The model under review builds one solid part; all positions refer to its coordinate system, in mm. Face numbers are marked on the shaded views. A direction names the side the tool comes from. Round coordinates to 2 decimals unless told otherwise and drop trailing zeros. Loops run counter-clockwise (first coordinate to the right, second up) from the corner with the lowest first, then second, coordinate; pieces in that order, holes last. Notation, with made-up numbers: M -27,0.5 L -1,0.5 A17 ccw -1,22.5 Z; hole C -36.5,-20.5 d11. An arc over 180 degrees is marked long. Answer as a JSON object with one key per item and string values. Group by question number.
Item 1: Tool access review of the marked faces 1 and 2: name each direction out of +Z, -Z, +X, -X, +Y, -Y from which nothing blocks a thin tool from reaching the whole face with its end or side.
Item 2: Consider section B-B (z = 7.5). Give the boundary of the cut face in (x, y) (3 decimals).
Item 3: To check wall thickness, follow line 1 (X direction, y = 139.7, z = 3.75) (3 decimals); line 2 (Y direction, x = 63, z = 5.25) (3 decimals); line 3 (Y direction, x = 69, z = 1.75) (3 decimals). State the ranges of each line that lie inside material, in increasing order.
Item 4: Consider section A-A (x = 63.5). Give the boundary of the cut face in (y, z) (3 decimals).
Item 5: Consider section D-D (y = 164.5). Give the boundary of the cut face in (x, z) (3 decimals), and give its area (3 significant figures).
Item 6: Consider section C-C (y = 139.7). Give the boundary of the cut face in (x, z) (3 decimals).
Item 7: Insertion check: P1, Ø6.5, axis at y = 128, z = 7.5, coming from the +X side (3 decimals); P2, Ø6.5, axis at x = 28.575, y = 76.2, coming from the -Z side. Each pin has a flat end and moves straight along its axis. Give the tip position at first contact, or say it passes through.
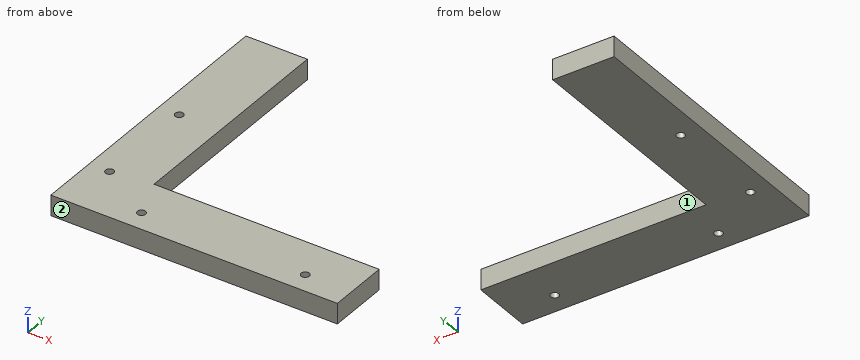
```python
from build123d import *

# Parameters (mm, degrees)
F1_DEPTH = 12.7
F2_D     = 5.08


with BuildPart() as f1:
    # F0 (on Top) → F1 (new body)
    with BuildSketch(Plane.XY):
        Polygon((193.675, 79.375), (53.975, 79.375), (53.975, 219.075), (15.875, 219.075), (15.875, 41.275), (193.675, 41.275), align=None)
    extrude(amount=F1_DEPTH)

    # F2 (through all)
    with Locations(Plane(origin=(0, 0, 0), x_dir=(1, 0, 0), z_dir=(0, 0, -1))):
        with Locations((28.575, -139.7), (28.575, -76.2), (63.5, -53.975), (165.1, -53.975)):
            Hole(F2_D / 2)


solid = f1.part
```
Geometry results:
{
 "1": {"face 1": "+Z, -Z, +X, +Y", "face 2": "+Z, -Z, +X, -X, -Y"},
 "2": {"outline": "M 15.875,41.275 L 193.675,41.275 L 193.675,79.375 L 53.975,79.375 L 53.975,219.075 L 15.875,219.075 Z; hole C 28.575,76.2 d5.08; hole C 28.575,139.7 d5.08; hole C 63.5,53.975 d5.08; hole C 165.1,53.975 d5.08"},
 "3": {"line 1": "x = 15.875 to 26.035, 31.115 to 53.975", "line 2": "y = 41.275 to 51.485, 56.465 to 79.375", "line 3": "y = 41.275 to 79.375"},
 "4": {"outline": "M 41.275,0 L 51.435,0 L 51.435,12.7 L 41.275,12.7 Z; M 56.515,0 L 79.375,0 L 79.375,12.7 L 56.515,12.7 Z"},
 "5": {"outline": "M 15.875,0 L 53.975,0 L 53.975,12.7 L 15.875,12.7 Z", "area": "484 mm^2"},
 "6": {"outline": "M 15.875,0 L 26.035,0 L 26.035,12.7 L 15.875,12.7 Z; M 31.115,0 L 53.975,0 L 53.975,12.7 L 31.115,12.7 Z"},
 "7": {"P1": "stops at x = 53.975", "P2": "stops at z = 0"}
}
